from build123d import *

# Parameters (mm, degrees)
F1_DEPTH = 140
F3_W     = 130
F3_H     = 80
F3_R     = 3
F4_DEPTH = 8
F6_W     = 80
F6_H     = 150
F6_R     = 2.5
F6_R_2   = 12.5
F7_DEPTH = 8


with BuildPart() as f1:
    # F0 (on Front) → F1 (new body)
    with BuildSketch(Plane.XZ):
        with BuildLine():
            ThreePointArc((40, 34), (38.2426406871, 38.2426406871), (34, 40))
            Line((34, 40), (-34, 40))
            ThreePointArc((-34, 40), (-38.2426406871, 38.2426406871), (-40, 34))
            Line((-40, 34), (-40, -34))
            ThreePointArc((-40, -34), (-38.2426406871, -38.2426406871), (-34, -40))
            Line((-34, -40), (34, -40))
            ThreePointArc((34, -40), (38.2426406871, -38.2426406871), (40, -34))
            Line((40, -34), (40, 34))
        make_face()
        with BuildLine():
            ThreePointArc((-36, 34), (-35.4142135624, 35.4142135624), (-34, 36))
            Line((-34, 36), (34, 36))
            ThreePointArc((34, 36), (35.4142135624, 35.4142135624), (36, 34))
            Line((36, 34), (36, -34))
            ThreePointArc((36, -34), (35.4142135624, -35.4142135624), (34, -36))
            Line((34, -36), (-34, -36))
            ThreePointArc((-34, -36), (-35.4142135624, -35.4142135624), (-36, -34))
            Line((-36, -34), (-36, 34))
        make_face(mode=Mode.SUBTRACT)
    extrude(amount=-F1_DEPTH)

    # F3 (on offset) → F4 (join)
    with BuildSketch(Plane.XZ.offset(8)):
        Rectangle(F3_W, F3_H)
        with Locations((-53, -28)):
            Circle(F3_R, mode=Mode.SUBTRACT)
        with Locations((53, -28)):
            Circle(F3_R, mode=Mode.SUBTRACT)
        with Locations((-53, 24)):
            Circle(F3_R, mode=Mode.SUBTRACT)
        with Locations((53, 24)):
            Circle(F3_R, mode=Mode.SUBTRACT)
    extrude(amount=-F4_DEPTH)

    # F6 (on offset) → F7 (join)
    with BuildSketch(Plane(origin=(0, 148, 0), x_dir=(-1, 0, 0), z_dir=(0, 1, 0))):
        with Locations((0, 35)):
            Rectangle(F6_W, F6_H)
        with Locations((-35, 30)):
            Circle(F6_R, mode=Mode.SUBTRACT)
        with Locations((35, 30)):
            Circle(F6_R, mode=Mode.SUBTRACT)
        with Locations((-35, 100)):
            Circle(F6_R, mode=Mode.SUBTRACT)
        with Locations((0, 65)):
            Circle(F6_R_2, mode=Mode.SUBTRACT)
        with Locations((35, 100)):
            Circle(F6_R, mode=Mode.SUBTRACT)
    extrude(amount=-F7_DEPTH)


solid = f1.part
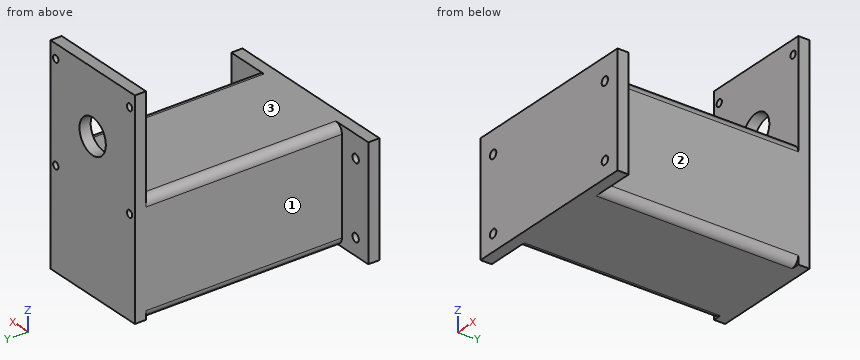
Check sheet for the modelled part. Datum: model origin and axes. Units: mm. Face numbers are marked on the shaded views. A direction names the side the tool comes from. Coordinates: 2 decimals unless noted, no trailing zeros. Write each loop counter-clockwise with the first axis right and the second up, starting at its lowest first coordinate (ties: lowest second). Pieces come first, ordered by that corner, then holes.
Item 1: Cross-section at C-C on y = 39.5. Record the boundary of the cut face in (x, z), then the cut area to 3 significant figures.
Numbers:
outline: (-40, -34) arc R6 ccw to (-34, -40) - (34, -40) arc R6 ccw to (40, -34) - (40, 34) arc R6 ccw to (34, 40) - (-34, 40) arc R6 ccw to (-40, 34) - close; hole (-36, -34) arc R2 ccw to (-34, -36) - (34, -36) arc R2 ccw to (36, -34) - (36, 34) arc R2 ccw to (34, 36) - (-34, 36) arc R2 ccw to (-36, 34) - close
area: 1,190 mm2
Item 2: Access from +Z, -Z, +X, -X, +Y, -Y to the whole of each face (thin tool, end or side, straight path). Record for the marked faces 1, 2 and 3.
Numbers:
face 1: +Z, -Z, -X, +Y
face 2: +Z, -Z, +X, +Y
face 3: +Z, +X, -X, -Y
Item 3: Cross-section at B-B on x = -53. Record the boundary of the cut face in (y, z), then the cut area to 3 significant figures.
Numbers:
outline: (-8, -40) - (0, -40) - (0, -31) - (-8, -31) - close; (-8, -25) - (0, -25) - (0, 21) - (-8, 21) - close; (-8, 27) - (0, 27) - (0, 40) - (-8, 40) - close
area: 544 mm2
Item 4: Cross-section at D-D on x = 0. Record the boundary of the cut face in (y, z).
Numbers:
outline: (-8, -40) - (148, -40) - (148, 52.5) - (140, 52.5) - (140, 40) - (-8, 40) - close; (140, 77.5) - (148, 77.5) - (148, 110) - (140, 110) - close; hole (0, -36) - (140, -36) - (140, 36) - (0, 36) - close
Item 5: Cross-section at A-A on z = 24. Record the boundary of the cut face in (x, y).
Numbers:
outline: (-65, -8) - (-56, -8) - (-56, 0) - (-65, 0) - close; (-50, -8) - (50, -8) - (50, 0) - (40, 0) - (40, 148) - (-40, 148) - (-40, 0) - (-50, 0) - close; (56, -8) - (65, -8) - (65, 0) - (56, 0) - close; hole (-36, 0) - (36, 0) - (36, 140) - (-36, 140) - close
Item 6: Scan lines: probe 1 along Z at (x, y) = (53, -1.75); probe 2 along Z at (x, y) = (-35, 144); probe 3 along X at (y, z) = (120.5, -18). Record each from-to range of solid material in increasing order.
Numbers:
probe 1: z = -40 to -31, -25 to 21, 27 to 40
probe 2: z = -40 to 27.5, 32.5 to 97.5, 102.5 to 110
probe 3: x = -40 to -36, 36 to 40
Item 7: Depth check by flat-ended pin: pin 1 Ø8 at (x, y) = (-39.5, 9) entering from +Z; pin 2 Ø1 at (x, y) = (38.5, 33.5) entering from -Z; pin 3 Ø20.5 at (y, z) = (86, 9.5) entering from -X. Enter the tip coordinate at first touch or a pass-through.
Numbers:
pin 1: stops at z = 39.81
pin 2: stops at z = -38.47
pin 3: stops at x = -40
